Part model, mm, in its own coordinate system. A direction names the side the tool comes from. Give positions to 0.01 mm unless a question says otherwise; leave off trailing zeros. Write each loop counter-clockwise with the first axis right and the second up, starting at its lowest first coordinate (ties: lowest second). Pieces come first, ordered by that corner, then holes.
from build123d import *

# Parameters (mm, degrees)
F0_R     = 11.43
F1_DEPTH = 5.08
F3_D     = 16.51
F5_DEPTH = 6.35
F6_R     = 1.84404


# Not quite as in the source:
# - a feature names something its author has since deleted; it is built from what else it names


with BuildPart() as f1:
    # F0 (on Front) → F1 (new body)
    with BuildSketch(Plane.XZ):
        Circle(F0_R)
    extrude(amount=F1_DEPTH)

    # F3 (through all)
    with Locations(Plane.XZ.offset(5.08)):
        with Locations((0, 0)):
            Hole(F3_D / 2)

    # F4 (on Front) → F5 (join)
    with BuildSketch(Plane.XZ):
        Polygon((-2.419047619, -2.419047619), (-2.54, 0), (-2.419047619, 2.419047619), (-12.7, 1.905), (-12.7, -1.905), align=None)
        Polygon((0, -2.54), (-2.419047619, -2.419047619), (-1.905, -12.7), (1.905, -12.7), (2.419047619, -2.419047619), align=None)
        Polygon((2.419047619, 2.419047619), (2.54, 0), (2.419047619, -2.419047619), (12.7, -1.905), (12.7, 1.905), align=None)
        Polygon((-1.905, 12.7), (-2.419047619, 2.419047619), (0, 2.54), (2.419047619, 2.419047619), (1.905, 12.7), align=None)
        Polygon((0, 0), (-2.54, 0), (-2.419047619, -2.419047619), (0, -2.54), align=None)
        Polygon((0, 2.54), (0, 0), (2.54, 0), (2.419047619, 2.419047619), align=None)
        Polygon((-2.419047619, 2.419047619), (-2.54, 0), (0, 0), (0, 2.54), align=None)
        Polygon((2.54, 0), (0, 0), (0, -2.54), (2.419047619, -2.419047619), align=None)
    extrude(amount=F5_DEPTH)

    # F6
    f6_edges = [f1.edges().sort_by_distance(p)[0] for p in [
        (-2.419048, -3.175, -2.419048),
        (-2.419048, -3.175, 2.419048),
        (2.419048, -3.175, 2.419048),
        (2.419048, -3.175, -2.419048),
        (-11.257705, -2.54, -1.977115),
        (-1.977115, -2.54, -11.257705),
        (1.977115, -2.54, -11.257705),
        (11.257705, -2.54, -1.977115),
        (11.257705, -2.54, 1.977115),
        (1.977115, -2.54, 11.257705),
        (-1.977115, -2.54, 11.257705),
        (-11.257705, -2.54, 1.977115),
        (7.972423, -2.54, 2.141379),
        (7.972423, -2.54, -2.141379),
        (2.141379, -2.54, -7.972423),
        (-2.141379, -2.54, -7.972423),
        (-7.972423, -2.54, -2.141379),
        (-7.972423, -2.54, 2.141379),
        (-2.141379, -2.54, 7.972423),
        (2.141379, -2.54, 7.972423),
    ]]
    fillet(f6_edges, radius=F6_R)


solid = f1.part
1) Saw through at D-D (y = -2). State how many separate pieces and enclosed holes the cut face has, and give its area (3 significant figures).
Check result:
separate pieces: 1
enclosed holes: 4
area: 372 mm2
2) Saw through at C-C (x = -9). Write the cut outline in (y, z), and give its area (3 significant figures).
Check result:
outline: (-6.35, -2.09) - (-5.08, -2.09) - (-5.08, -7.05) - (0, -7.05) - (0, 7.05) - (-5.08, 7.05) - (-5.08, 2.09) - (-6.35, 2.09) - close
area: 76.9 mm2
3) Drill centre lines: L1, parallel to Z at x = -5.5, y = -3.5; L2, parallel to Z at x = 3.5, y = -1.5; L3, parallel to X at y = -4, z = -5. Where is each one in solid material? Low to high.
Check result:
L1: z = -10.02 to -6.16, -2.4 to 2.4, 6.16 to 10.02
L2: z = -10.88 to -6.62, -2.46 to 2.46, 6.62 to 10.88
L3: x = -10.28 to -6.53, -2.3 to 2.3, 6.53 to 10.28
4) Mould opens along X. For faces 1 (the flat face through (12.7, -3, 0)), 2 (the flat face through (0, -3, 12.7)), 3 (the cylindrical face through (-8.138, -2.504, -8.026)), 4 (the flat face through (2.167, -5.277, -7.456)) say: +X half, -X half, draft (parallel to the pull), parting line (faces both ways), or undercut.
Check result:
face 1: +X half
face 2: draft
face 3: -X half
face 4: undercut
5) Flat gauge pins, fed straight in: P1, Ø3, axis at y = -4.5, z = -8.5, coming from the -X side; P2, Ø8.5, axis at x = -9, z = -7, coming from the -Y side; P3, Ø2, axis at x = 5.5, y = -5.5, coming from the -Z side. Where does each tip first touch, or does it go through?
Check result:
P1: stops at x = -9.04
P2: stops at y = -5.08
P3: stops at z = -10.47
6) 3-axis set-ups, long thin cutter, end or side, ignore diameter. For faces 5 (the flat face through (7.456, -5.277, 2.167)), 6 (the flat face through (-6, -5.08, 6)), 7 (the cylindrical face through (6.56, -2.5, -3.35)): which of +Z, -Z, +X, -X, +Y, -Y reach the whole face in a straight line?
Check result:
face 5: -Y
face 6: +Z, -X, -Y
face 7: +Y, -Y
7) Saw through at B-B (z = 10.5). Write the cut outline in (x, y) (3 decimals).
Check result:
outline: (-4.516, -5.08) - (-2.015, -5.08) - (-2.015, -6.35) - (2.015, -6.35) - (2.015, -5.08) - (4.516, -5.08) - (4.516, 0) - (-4.516, 0) - close
8) Saw through at A-A (x = -6). Write the cut outline in (y, z), and give its area (3 significant figures).
Check result:
outline: (-6.35, -2.24) - (-5.08, -2.24) - (-5.08, -2.67) - (0, -2.67) - (0, 2.67) - (-5.08, 2.67) - (-5.08, 2.24) - (-6.35, 2.24) - close; (-5.08, -9.73) - (0, -9.73) - (0, -5.67) - (-5.08, -5.67) - close; (-5.08, 5.67) - (0, 5.67) - (0, 9.73) - (-5.08, 9.73) - close
area: 74.0 mm2
